```python
from build123d import *

# Parameters (mm, degrees)
EXTRUDE_1_DEPTH     = 0.25
EXTRUDE_1_2_DEPTH   = 0.25
CUT_EXTRUDE_1_REACH = 10.99


with BuildPart() as part:
    # Sketch 1 → Extrude 1 (new, symmetric)
    with BuildSketch(Plane.XZ):
        Polygon((-1.52, 3.6), (-1.52, 1), (-1.62, 1), (-1.62, 0), (-1.52, 0), (-1.52, -3), (-1.02, -3), (-1.02, 0), (-0.92, 0), (-0.92, 1), (-1.02, 1), (-1.02, 3.6), align=None)
    extrude(amount=EXTRUDE_1_DEPTH, both=True)



with BuildPart() as body_2:
    # Sketch 1 → Extrude 1 2 (new, symmetric)
    with BuildSketch(Plane.XZ):
        Polygon((1.02, 3.6), (1.02, 1), (0.92, 1), (0.92, 0), (1.02, 0), (1.02, -3), (1.52, -3), (1.52, 0), (1.62, 0), (1.62, 1), (1.52, 1), (1.52, 3.6), align=None)
    extrude(amount=EXTRUDE_1_2_DEPTH, both=True)


with BuildPart() as part_1:
    add(part.part)

    add(body_2.part)  # Revolve 1 merges body 2
    # Sketch 2 → Revolve 1 (revolve)
    with BuildSketch(Plane(origin=(0, 0, 0), x_dir=(1, 0, 0), z_dir=(0, 1, 0))):
        with BuildLine():
            Line((0, -3.6), (0, -12.6))
            ThreePointArc((0, -12.6), (1.767766953, -11.867766953), (2.5, -10.1))
            Line((2.5, -10.1), (2.5, -4.6))
            Line((2.5, -4.6), (2.9, -4.6))
            Line((2.9, -4.6), (2.9, -3.6))
            Line((2.9, -3.6), (0, -3.6))
        make_face()
    revolve(axis=Axis((0, 0, 3.6), (0, 0, -1)))

    # Sketch 3 → Cut-Extrude 1 (cut, up to next)
    with BuildSketch(Plane.XY.offset(4.6), mode=Mode.PRIVATE) as cut_extrude_1_sk1:
        with BuildLine():
            Line((2.5, 1.469693846), (2.5, -1.469693846))
            ThreePointArc((2.5, -1.469693846), (2.9, 0), (2.5, 1.469693846))
        make_face()
    cut_extrude_1_tool1 = extrude(cut_extrude_1_sk1.sketch, amount=-CUT_EXTRUDE_1_REACH, mode=Mode.PRIVATE) & part_1.part
    add(cut_extrude_1_tool1.solids().sort_by_distance((2.660985, 0, 4.6))[0], mode=Mode.SUBTRACT)


solid = part_1.part
```
Can you work these out from the model? Positions are in its coordinate system, mm. A direction names the side the tool comes from. Coordinates: 2 decimals unless noted, no trailing zeros. Loops run counter-clockwise (first coordinate to the right, second up) from the corner with the lowest first, then second, coordinate; pieces in that order, holes last. Notation, with made-up numbers: (-13, 68) -> (45, 68) arc R13 ccw to (45, 75) -> close; hole circle Ø11 at (62, -13). An arc over 180 degrees is marked (long way). Put each result on its own line as item: value. Start each with the question number.
Q1. I'm going to push flat-ended pins straight in: P1, Ø0.6, axis at y = 0, z = -1.5, coming from the +X side; P2, Ø1, axis at x = -1, z = 7.5, coming from the -Y side; P3, Ø0.6, axis at y = 0, z = 0.5, coming from the -X side. Where does each tip first touch, or does it pass through?
Q2. I want a section at A-A (x = 0). Write out the boundary of the cut face in (y, z).
Q3. I want a section at B-B (y = -2). Write out the boundary of the cut face in (x, z), plus the area to 3 significant figures.
Q4. For faces 1 (the face through (-0.54, 2.44, 7.31)), 2 (the face through (-2.9, -0.1, 4.1)), which set-ups out of +Z, -Z, +X, -X, +Y, -Y let a thin tool reach every point of the face, with its end or its side?
Q5. I want a section at C-C (z = 9). Write out the boundary of the cut face in (x, y), plus the area to 3 significant figures.
Q6. I want a section at D-D (z = 11.25). Write out the boundary of the cut face in (x, y).
Q7. If I drill on line 1 (Z direction, x = -1.25, y = 2.4); line 2 (X direction, y = -0.2, z = 11.5); line 3 (Z direction, x = -1.4, y = 1.05), over which ranges is the centre line in solid material (lowest first)? Write a range as [from, to].
Taken from the geometry:
1. P1: stops at x = 1.52
1. P2: stops at y = -2.45
1. P3: stops at x = -1.62
2. outline: (-2.9, 3.6) -> (2.9, 3.6) -> (2.9, 4.6) -> (2.5, 4.6) -> (2.5, 10.1) arc R2.5 ccw to (-2.5, 10.1) -> (-2.5, 4.6) -> (-2.9, 4.6) -> close
3. outline: (-2.1, 3.6) -> (2.1, 3.6) -> (2.1, 4.6) -> (1.5, 4.6) -> (1.5, 10.1) arc R1.5 ccw to (-1.5, 10.1) -> (-1.5, 4.6) -> (-2.1, 4.6) -> close
3. area: 24.2 mm2
4. face 1: +Z
4. face 2: +Z, -Z
5. outline: circle Ø5 at (0, 0)
5. area: 19.6 mm2
6. outline: circle Ø4.44 at (0, 0)
7. line 1: z = [3.6, 4.6]
7. line 2: x = [-2.06, 2.06]
7. line 3: z = [3.6, 11.89]
